Can you work these out from the model? Positions are in its coordinate system, mm. Face numbers are marked on the shaded views. A direction names the side the tool comes from. Give positions to 0.01 mm unless a question says otherwise; leave off trailing zeros. Loops run counter-clockwise (first coordinate to the right, second up) from the corner with the lowest first, then second, coordinate; pieces in that order, holes last. Notation, with made-up numbers: M 51,3 L 101,3 A7 ccw 101,11 Z; hole C 17.25,85 d9. An arc over 180 degrees is marked long. Put each result on its own line as item: value. Start each with the question number.
1) Please list where these lines run through material, in increasing order: line 1 along Y through (x, z) = (-4, 9.5) (3 decimals); line 2 along X through (y, z) = (111, -1.5); line 3 along Z through (x, y) = (12.5, 103). Write a range as from..to.
2) Imagine slicing it at A-A (y = 71). Write out the boundary of the cut face in (x, z) (1 decimal), then the cut area to 3 significant figures.
3) For the marked faces 1 and 2, which set-ups out of +Z, -Z, +X, -X, +Y, -Y let a thin tool reach every point of the face, with its end or its side?
4) For P1, Ø2, axis at x = 19.5, y = 48, coming from the -Z side; P2, Ø1.5, axis at y = 145, z = -20, coming from the +X side; P3, Ø6, axis at y = 149, z = 14, coming from the +X side, each with a flat end and sliding along its axis, tell me the tip position at first contact or that it passes through.
from build123d import *

# Parameters (mm, degrees)
FILLET1_R = 2.54
FILLET2_R = 0.635
FILLET3_R = 6.35


with BuildPart() as part:
    # Sketch2 → Revolve1 (revolve)
    with BuildSketch(Plane.XY, mode=Mode.PRIVATE) as revolve1_sk:
        with BuildLine():
            Line((32.0675, 0), (32.0675, 195.58))
            ThreePointArc((32.0675, 195.58), (26.829595401, 213.144093113), (12.827, 224.97034922))
            Line((12.827, 224.97034922), (12.827, 238.125))
            Line((12.827, 238.125), (0, 238.125))
            Line((0, 238.125), (0, 0.889))
            Line((0, 0.889), (23.114, 0.889))
            Line((23.114, 0.889), (23.114, 0))
            Line((23.114, 0), (32.0675, 0))
        make_face()
    revolve(revolve1_sk.sketch.rotate(Axis((0, 238.125, 0), (0, -1, 0)), 180), axis=Axis((0, 238.125, 0), (0, -1, 0)))

    # Fillet1
    # the kernel refuses this fillet: 2.54 mm, written as the material it adds along each edge
    with BuildSketch(Plane(origin=(0, 0.889, 0), x_dir=(-1, 0, 0), z_dir=(0, 0, 1))) as fillet1_piece_1:
        with BuildLine():
            CenterArc((21.183767112, 2.54), FILLET1_R, 270, 49.458398126)
            Line((23.114, 0.889), (23.114, 0))
            Line((23.114, 0), (21.183767112, 0))
        make_face()
    revolve(axis=Axis((0, 0.889, 0), (0, -1, 0)))
    # the kernel refuses this fillet: 2.54 mm, written as the material it takes off along each edge
    with BuildSketch(Plane(origin=(0, 0, 0), x_dir=(-1, 0, 0), z_dir=(0, 0, 1))) as fillet1_2_piece_1:
        with BuildLine():
            CenterArc((32.0675 - FILLET1_R, -FILLET1_R), FILLET1_R, 0, 90)
            Line((32.0675 - FILLET1_R, 0), (32.0675, 0))
            Line((32.0675, 0), (32.0675, -FILLET1_R))
        make_face()
    revolve(axis=Axis((0, 0, 0), (0, -1, 0)), mode=Mode.SUBTRACT)

    # Fillet2
    fillet2_edges = [part.edges().sort_by_distance(p)[0] for p in [
        (12.827, 238.125, 0),
    ]]
    fillet(fillet2_edges, radius=FILLET2_R)

    # Fillet3
    fillet3_edges = [part.edges().sort_by_distance(p)[0] for p in [
        (12.827, 224.97034922, 0),
    ]]
    fillet(fillet3_edges, radius=FILLET3_R)


solid = part.part
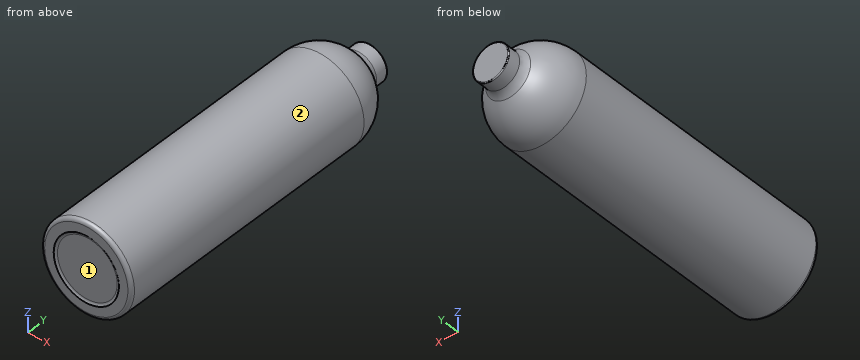
Recorded:
1. line 1: 0.889..238.125
1. line 2: -32.03..32.03
1. line 3: -29.53..29.53
2. outline: C 0,0 d64.1
2. area: 3,230 mm²
3. face 1: -Y
3. face 2: +Y, -Y
4. P1: z = -26.19
4. P2: x = 25.65
4. P3: x = 30.12
